Here's how the part is built. I have some questions about the finished solid (model axes, mm). Face numbers are marked on the shaded views. A direction names the side the tool comes from. Coordinates: 2 decimals unless noted, no trailing zeros. Loops run counter-clockwise (first coordinate to the right, second up) from the corner with the lowest first, then second, coordinate; pieces in that order, holes last. Notation, with made-up numbers: (50.25, -20.5) -> (71.25, -20.5) arc R14 cw to (71.25, -14.5) -> close; hole circle Ø9 at (-38.5, 47). An arc over 180 degrees is marked (long way). Answer as a JSON object with one key per item and string values. Group by question number.
Q1. I want a section at A-A on y = 1.75. Write out the boundary of the cut face in (x, z) (3 decimals), then the cut area to 3 significant figures.
Q2. I'm going to push flat-ended pins straight in: pin 1 (3 mm diameter, centred on y = 12.5, z = 0.5, fed in from -X) (3 decimals); pin 2 (1.5 mm diameter, centred on x = -5, z = -1.5, fed in from +Y); pin 3 (3.5 mm diameter, centred on x = 5, z = -3, fed in from +Y); pin 4 (5 mm diameter, centred on x = -5, z = -2.5, fed in from -Y). Where does each tip first touch, or does it pass through?
Q3. On a 3-axis mill with a long thin cutter (end or side, diameter ignored), from which of +Z, -Z, +X, -X, +Y, -Y can I reach the whole of each face in a straight line? I mean the marked faces 1, 2, 3 and 4. Say none if no direction works.
Q4. I need wall thicknesses on line 1 (Y direction, x = -5.75, z = 3); line 2 (X direction, y = 4.5, z = 0) (3 decimals); line 3 (X direction, y = 12.75, z = 1). Which ranges of each line are inside material? Lowest first, please.
Q5. I want a section at B-B on x = 5.5. Write out the boundary of the cut face in (y, z), then the cut area to 3 significant figures.
Q6. I want a section at D-D on y = 9. Write out the boundary of the cut face in (x, z) (3 decimals), then the cut area to 3 significant figures.
Q7. I want a section at C-C on y = -0.5. Write out the boundary of the cut face in (x, z) (3 decimals).
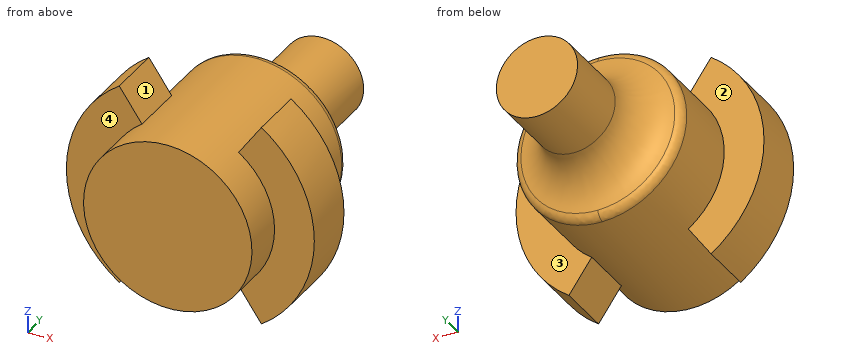
```python
from build123d import *

# Parameters (mm, degrees)
SALIENTE_EXTRUIR1_START   = 0.4
SALIENTE_EXTRUIR1_DEPTH   = 3.15
SALIENTE_EXTRUIR1_2_DEPTH = 3.15
CROQUIS1_3_R              = 4.925
SALIENTE_EXTRUIR2_DEPTH   = 8
SALIENTE_EXTRUIR3_START   = -2
CROQUIS1_4_R              = 4.925
SALIENTE_EXTRUIR3_DEPTH   = 2
CROQUIS2_R                = 2.375
SALIENTE_EXTRUIR4_DEPTH   = 6.5
REDONDEO2_R               = 2.5
REDONDEO3_R               = 0.5


with BuildPart() as part:
    # Croquis1 → Saliente-Extruir1 (new body)
    with BuildSketch(Plane(origin=(0, 0, 0), x_dir=(1, 0, 0), z_dir=(0, 1, 0)).offset(SALIENTE_EXTRUIR1_START)):
        with BuildLine():
            ThreePointArc((-2.824863949, -4.034323818), (-4.925, 0), (-2.824863949, 4.034323818))
            Line((-2.824863949, 4.034323818), (-4.158429164, 5.938852321))
            ThreePointArc((-4.158429164, 5.938852321), (-7.25, 0), (-4.158429164, -5.938852321))
            Line((-4.158429164, -5.938852321), (-2.824863949, -4.034323818))
        make_face()
    extrude(amount=SALIENTE_EXTRUIR1_DEPTH)



with BuildPart() as body_2:
    # Croquis1 → Saliente-Extruir1 2 (new body)
    with BuildSketch(Plane(origin=(0, 0, 0), x_dir=(1, 0, 0), z_dir=(0, 1, 0)).offset(SALIENTE_EXTRUIR1_START)):
        with BuildLine():
            Line((4.158429164, 5.938852321), (2.824863949, 4.034323818))
            ThreePointArc((2.824863949, 4.034323818), (4.368528353, 2.27411192), (4.925, 0))
            ThreePointArc((4.925, 0), (4.368528353, -2.27411192), (2.824863949, -4.034323818))
            Line((2.824863949, -4.034323818), (4.158429164, -5.938852321))
            ThreePointArc((4.158429164, -5.938852321), (7.25, 0), (4.158429164, 5.938852321))
        make_face()
    extrude(amount=SALIENTE_EXTRUIR1_2_DEPTH)


with BuildPart() as part_1:
    add(part.part)

    add(body_2.part)  # Saliente-Extruir2 merges body 2
    # Croquis1_3 → Saliente-Extruir2 (add)
    with BuildSketch(Plane(origin=(0, 0, 0), x_dir=(1, 0, 0), z_dir=(0, 1, 0))):
        with Locations(Location((0, 0, 0), (0, 0, 270))):
            Circle(CROQUIS1_3_R)
    extrude(amount=SALIENTE_EXTRUIR2_DEPTH)

    # Croquis1_4 → Saliente-Extruir3 (add)
    with BuildSketch(Plane(origin=(0, 0, 0), x_dir=(1, 0, 0), z_dir=(0, 1, 0)).offset(SALIENTE_EXTRUIR3_START)):
        with Locations(Location((0, 0, 0), (0, 0, 270))):
            Circle(CROQUIS1_4_R)
    extrude(amount=SALIENTE_EXTRUIR3_DEPTH)

    # Croquis2 → Saliente-Extruir4 (add)
    with BuildSketch(Plane(origin=(0, 8, 0), x_dir=(1, 0, 0), z_dir=(0, 1, 0))):
        with Locations(Location((0, 0, 0), (0, 0, 90))):
            Circle(CROQUIS2_R)
    extrude(amount=SALIENTE_EXTRUIR4_DEPTH)

    # Redondeo2
    redondeo2_edges = [part_1.edges().sort_by_distance(p)[0] for p in [
        (0, 8, 2.375),
    ]]
    fillet(redondeo2_edges, radius=REDONDEO2_R)

    # Redondeo3
    redondeo3_edges = [part_1.edges().sort_by_distance(p)[0] for p in [
        (0, 8, -4.925),
    ]]
    fillet(redondeo3_edges, radius=REDONDEO3_R)


solid = part_1.part
```
Result set:
{
 "1": {"outline": "(-4.158, -5.939) -> (-2.825, -4.034) arc R4.925 ccw to (2.825, -4.034) -> (4.158, -5.939) arc R7.25 ccw to (4.158, 5.939) -> (2.825, 4.034) arc R4.925 ccw to (-2.825, 4.034) -> (-4.158, 5.939) arc R7.25 ccw to start", "area": "131 mm²"},
 "2": {"pin 1": "stops at x = -2.375", "pin 2": "stops at y = 8.03", "pin 3": "stops at y = 8.13", "pin 4": "stops at y = -2"},
 "3": {"face 1": "+Z, +Y, -Y", "face 2": "-X, +Y", "face 3": "+X, +Y", "face 4": "-X, -Y"},
 "4": {"line 1": "y = 0.4 to 3.55", "line 2": "x = -4.925 to 4.925", "line 3": "x = -2.15 to 2.15"},
 "5": {"outline": "(0.4, -4.72) -> (3.55, -4.72) -> (3.55, 4.72) -> (0.4, 4.72) -> close", "area": "29.8 mm²"},
 "6": {"outline": "circle Ø5.75 at (0, 0)", "area": "26.0 mm²"},
 "7": {"outline": "circle Ø9.85 at (0, 0)"}
}
